Input: part model. Units: mm. Frame: model coordinates. A direction names the side the tool comes from. Give positions to 0.01 mm unless a question says otherwise; leave off trailing zeros. Loops run counter-clockwise (first coordinate to the right, second up) from the corner with the lowest first, then second, coordinate; pieces in that order, holes last. Notation, with made-up numbers: (51.5, 7) - (93.5, 7) arc R22 cw to (93.5, 30) - close; hole circle Ø8 at (27.25, 57). An arc over 180 degrees is marked (long way). Answer as a JSON object with one key per item and string values. Group by question number.
(1) Mould query, pull axis Z, two halves, no side actions, for faces 1 (the flat face through (0, 8, 9)), 2 (the flat face through (0, 2, -25.981)), 3 (the cylindrical face through (1.008, 1.423, 31.078)). Classes: +Z half, -Z half, draft (parallel to the pull), parting line (faces both ways), or undercut.
(2) Section query B-B (z = 17). Return loops of the section in (x, y), plus the area to 3 significant figures.
(3) Pin query (flat end, axial travel): P1, Ø2, axis at y = 3.5, z = -14, coming from the -X side; P2, Ø2, axis at y = 1.5, z = -8.5, coming from the -X side; P3, Ø4, axis at x = -30.5, y = 4.5, coming from the +Z side; P4, Ø4, axis at y = 1, z = -10.5, coming from the +X side. Return the tip coordinate at first contact, or that it passes through.
(4) Access query for faces 4 (the cylindrical face through (-22.624, 4.056, -13.77)), 5 (the cylindrical face through (-6.967, 6.768, 4.229)). Directions: +Z, -Z, +X, -X, +Y, -Y. A direction counts if a zero-diameter tool reaches every point of the face in a straight line with its end or side. Return the directions, or none.
(5) Material intervals for L1, parallel to Z at x = -27.5, y = 3.5; L2, parallel to X at y = 3, z = 9; L3, parallel to Z at x = 17, y = 3.5, sorted ascending.
(6) Section query A-A (z = 0). Return loops of the section in (x, y), plus the area to 3 significant figures.
```python
from build123d import *

# Parameters (mm, degrees)
BOSS_EXTRUDE1_DEPTH   = 8
CHAMFER1_SIZE         = 4
CHAMFER1_SIZE2        = 6.928203
CHAMFER1_PART_2_SIZE  = 4
CHAMFER1_PART_2_SIZE2 = 6.928203
CHAMFER1_PART_3_SIZE  = 4
CHAMFER1_PART_3_SIZE2 = 6.928203
CUT_EXTRUDE1_REACH    = 61.292
SKETCH2_R             = 1.6
CUT_EXTRUDE2_REACH    = 67.292
CUT_EXTRUDE2_START    = -6
SKETCH3_R             = 3
CIRPATTERN1_COUNT     = 3
CUT_EXTRUDE4_DEPTH    = 2.5
CUT_EXTRUDE5_REACH    = 57.633
SKETCH10_R            = 1.6


with BuildPart() as part:
    # Sketch1 → Boss-Extrude1 (new body)
    with BuildSketch(Plane(origin=(0, 0, 0), x_dir=(1, 0, 0), z_dir=(0, 1, 0))):
        Polygon((-31, 25.980762), (31, 25.980762), (38, 13.856406), (7, -39.837169), (-7, -39.837169), (-38, 13.856406), align=None)
        with BuildLine():
            Line((3.923683, -4.605129), (5.655734, -3.605129))
            ThreePointArc((5.655734, -3.605129), (14.562222, 8.407503), (-0.294266, 6.700574))
            Line((-0.294266, 6.700574), (-2.026317, 5.700574))
            ThreePointArc((-2.026317, 5.700574), (-5.239454, -3.025), (3.923683, -4.605129))
        make_face(mode=Mode.SUBTRACT)
    extrude(amount=BOSS_EXTRUDE1_DEPTH)

    # Chamfer1
    chamfer1_edges = [part.edges().sort_by_distance(p)[0] for p in [
        (22.5, 8, 12.990381),
    ]]
    chamfer1_side = [part.faces().sort_by_distance(p)[0] for p in [
        (22.5, 4, 12.990381),
    ]]
    chamfer(chamfer1_edges, length=CHAMFER1_SIZE, length2=CHAMFER1_SIZE2, reference=chamfer1_side[0])

    # Chamfer1 part 2
    chamfer1_part_2_edges = [part.edges().sort_by_distance(p)[0] for p in [
        (-22.5, 8, 12.990381),
    ]]
    chamfer1_part_2_side = [part.faces().sort_by_distance(p)[0] for p in [
        (-22.5, 4, 12.990381),
    ]]
    chamfer(chamfer1_part_2_edges, length=CHAMFER1_PART_2_SIZE, length2=CHAMFER1_PART_2_SIZE2, reference=chamfer1_part_2_side[0])

    # Chamfer1 part 3
    chamfer1_part_3_edges = [part.edges().sort_by_distance(p)[0] for p in [
        (0, 8, -25.980762),
    ]]
    chamfer1_part_3_side = [part.faces().sort_by_distance(p)[0] for p in [
        (0, 4, -25.980762),
    ]]
    chamfer(chamfer1_part_3_edges, length=CHAMFER1_PART_3_SIZE, length2=CHAMFER1_PART_3_SIZE2, reference=chamfer1_part_3_side[0])

    # Cut-Extrude1: up to this plane
    cut_extrude1_end = Plane(origin=(0, 0, 0), z_dir=(0, -1, 0))
    # Sketch2 → Cut-Extrude1 (cut, up to the surface)
    with BuildSketch(Plane(origin=(7.125, 14.25, 4.113621), x_dir=(0.9013878188659966, -0.41602514716892336, -0.12009611535381544), z_dir=(0.43301270189222085, 0.8660254037844383, 0.24999999999999917)), mode=Mode.PRIVATE) as cut_extrude1_sk1:
        with Locations(Location((28.428385, 12.89678, 0), (0, 0, 172.874984))):
            Circle(SKETCH2_R)
    cut_extrude1_tool1 = split(extrude(cut_extrude1_sk1.sketch, amount=-CUT_EXTRUDE1_REACH, mode=Mode.PRIVATE), bisect_by=cut_extrude1_end, keep=Keep.BOTH, mode=Mode.PRIVATE)
    # Sketch2 → Cut-Extrude1 (cut, up to the surface)
    with BuildSketch(Plane(origin=(7.125, 14.25, 4.113621), x_dir=(0.9013878188659966, -0.41602514716892336, -0.12009611535381544), z_dir=(0.43301270189222085, 0.8660254037844383, 0.24999999999999917)), mode=Mode.PRIVATE) as cut_extrude1_sk2:
        with Locations(Location((-0.970725, -31.201886, 0), (0, 0, 172.874984))):
            Circle(SKETCH2_R)
    cut_extrude1_tool2 = split(extrude(cut_extrude1_sk2.sketch, amount=-CUT_EXTRUDE1_REACH, mode=Mode.PRIVATE), bisect_by=cut_extrude1_end, keep=Keep.BOTH, mode=Mode.PRIVATE)
    # Sketch2 → Cut-Extrude1 (cut, up to the surface)
    with BuildSketch(Plane(origin=(7.125, 14.25, 4.113621), x_dir=(0.9013878188659966, -0.41602514716892336, -0.12009611535381544), z_dir=(0.43301270189222085, 0.8660254037844383, 0.24999999999999917)), mode=Mode.PRIVATE) as cut_extrude1_sk3:
        with Locations(Location((13.72883, -9.152553, 0), (0, 0, 172.874984))):
            Circle(SKETCH2_R)
    cut_extrude1_tool3 = split(extrude(cut_extrude1_sk3.sketch, amount=-CUT_EXTRUDE1_REACH, mode=Mode.PRIVATE), bisect_by=cut_extrude1_end, keep=Keep.BOTH, mode=Mode.PRIVATE)
    # Sketch2 → Cut-Extrude1 (cut, up to the surface)
    with BuildSketch(Plane(origin=(7.125, 14.25, 4.113621), x_dir=(0.9013878188659966, -0.41602514716892336, -0.12009611535381544), z_dir=(0.43301270189222085, 0.8660254037844383, 0.24999999999999917)), mode=Mode.PRIVATE) as cut_extrude1_sk4:
        with Locations(Location((22.881383, 4.576277, 0), (0, 0, 172.874984))):
            Circle(SKETCH2_R)
    cut_extrude1_tool4 = split(extrude(cut_extrude1_sk4.sketch, amount=-CUT_EXTRUDE1_REACH, mode=Mode.PRIVATE), bisect_by=cut_extrude1_end, keep=Keep.BOTH, mode=Mode.PRIVATE)
    # Sketch2 → Cut-Extrude1 (cut, up to the surface)
    with BuildSketch(Plane(origin=(7.125, 14.25, 4.113621), x_dir=(0.9013878188659966, -0.41602514716892336, -0.12009611535381544), z_dir=(0.43301270189222085, 0.8660254037844383, 0.24999999999999917)), mode=Mode.PRIVATE) as cut_extrude1_sk5:
        with Locations(Location((4.576277, -22.881383, 0), (0, 0, 172.874984))):
            Circle(SKETCH2_R)
    cut_extrude1_tool5 = split(extrude(cut_extrude1_sk5.sketch, amount=-CUT_EXTRUDE1_REACH, mode=Mode.PRIVATE), bisect_by=cut_extrude1_end, keep=Keep.BOTH, mode=Mode.PRIVATE)
    cut_extrude1 = cut_extrude1_tool1.solids().sort_by_distance((32.75, 6, -11.691343))[0] + cut_extrude1_tool2.solids().sort_by_distance((6.25, 6, 34.208003))[0] + cut_extrude1_tool3.solids().sort_by_distance((19.5, 6, 11.25833))[0] + cut_extrude1_tool4.solids().sort_by_distance((27.75, 6, -3.031089))[0] + cut_extrude1_tool5.solids().sort_by_distance((11.25, 6, 25.547749))[0]
    add(cut_extrude1, mode=Mode.SUBTRACT)

    # Sketch3 → Cut-Extrude2 (cut, up to next)
    with BuildSketch(Plane(origin=(7.125, 14.25, 4.113621), x_dir=(0.9013878188659967, -0.41602514716892325, -0.12009611535381544), z_dir=(0.43301270189222074, 0.8660254037844383, 0.24999999999999925)).offset(CUT_EXTRUDE2_START), mode=Mode.PRIVATE) as cut_extrude2_sk1:
        with Locations((28.428385, 12.89678)):
            Circle(SKETCH3_R)
    cut_extrude2_tool1 = extrude(cut_extrude2_sk1.sketch, amount=-CUT_EXTRUDE2_REACH, mode=Mode.PRIVATE) & part.part
    # Sketch3 → Cut-Extrude2 (cut, up to next)
    with BuildSketch(Plane(origin=(7.125, 14.25, 4.113621), x_dir=(0.9013878188659967, -0.41602514716892325, -0.12009611535381544), z_dir=(0.43301270189222074, 0.8660254037844383, 0.24999999999999925)).offset(CUT_EXTRUDE2_START), mode=Mode.PRIVATE) as cut_extrude2_sk2:
        with Locations((-0.970725, -31.201886)):
            Circle(SKETCH3_R)
    cut_extrude2_tool2 = extrude(cut_extrude2_sk2.sketch, amount=-CUT_EXTRUDE2_REACH, mode=Mode.PRIVATE) & part.part
    # Sketch3 → Cut-Extrude2 (cut, up to next)
    with BuildSketch(Plane(origin=(7.125, 14.25, 4.113621), x_dir=(0.9013878188659967, -0.41602514716892325, -0.12009611535381544), z_dir=(0.43301270189222074, 0.8660254037844383, 0.24999999999999925)).offset(CUT_EXTRUDE2_START), mode=Mode.PRIVATE) as cut_extrude2_sk3:
        with Locations((13.72883, -9.152553)):
            Circle(SKETCH3_R)
    cut_extrude2_tool3 = extrude(cut_extrude2_sk3.sketch, amount=-CUT_EXTRUDE2_REACH, mode=Mode.PRIVATE) & part.part
    # Sketch3 → Cut-Extrude2 (cut, up to next)
    with BuildSketch(Plane(origin=(7.125, 14.25, 4.113621), x_dir=(0.9013878188659967, -0.41602514716892325, -0.12009611535381544), z_dir=(0.43301270189222074, 0.8660254037844383, 0.24999999999999925)).offset(CUT_EXTRUDE2_START), mode=Mode.PRIVATE) as cut_extrude2_sk4:
        with Locations((22.881383, 4.576277)):
            Circle(SKETCH3_R)
    cut_extrude2_tool4 = extrude(cut_extrude2_sk4.sketch, amount=-CUT_EXTRUDE2_REACH, mode=Mode.PRIVATE) & part.part
    # Sketch3 → Cut-Extrude2 (cut, up to next)
    with BuildSketch(Plane(origin=(7.125, 14.25, 4.113621), x_dir=(0.9013878188659967, -0.41602514716892325, -0.12009611535381544), z_dir=(0.43301270189222074, 0.8660254037844383, 0.24999999999999925)).offset(CUT_EXTRUDE2_START), mode=Mode.PRIVATE) as cut_extrude2_sk5:
        with Locations((4.576277, -22.881383)):
            Circle(SKETCH3_R)
    cut_extrude2_tool5 = extrude(cut_extrude2_sk5.sketch, amount=-CUT_EXTRUDE2_REACH, mode=Mode.PRIVATE) & part.part
    cut_extrude2_1 = cut_extrude2_tool1.solids().sort_by_distance((30.151924, 0.803848, -13.191343))[0]
    add(cut_extrude2_1, mode=Mode.SUBTRACT)
    cut_extrude2_2 = cut_extrude2_tool2.solids().sort_by_distance((3.651924, 0.803848, 32.708003))[0]
    add(cut_extrude2_2, mode=Mode.SUBTRACT)
    cut_extrude2_3 = cut_extrude2_tool3.solids().sort_by_distance((16.901924, 0.803848, 9.75833))[0]
    add(cut_extrude2_3, mode=Mode.SUBTRACT)
    cut_extrude2_4 = cut_extrude2_tool4.solids().sort_by_distance((25.151924, 0.803848, -4.531089))[0]
    add(cut_extrude2_4, mode=Mode.SUBTRACT)
    cut_extrude2_5 = cut_extrude2_tool5.solids().sort_by_distance((8.651924, 0.803848, 24.047749))[0]
    add(cut_extrude2_5, mode=Mode.SUBTRACT)
    cut_extrude2 = cut_extrude2_1 + cut_extrude2_2 + cut_extrude2_3 + cut_extrude2_4 + cut_extrude2_5  # Cut-Extrude2 as one shape, for the pattern or mirror that repeats it

    # CirPattern1: Cut-Extrude1, Cut-Extrude2 ×3 about axis
    cirpattern1_axis = Axis((0, 0, 0), (0, 1, 0))
    add([cut_extrude1.rotate(cirpattern1_axis, i * 360 / CIRPATTERN1_COUNT) for i in range(1, CIRPATTERN1_COUNT)], mode=Mode.SUBTRACT)
    add([cut_extrude2.rotate(cirpattern1_axis, i * 360 / CIRPATTERN1_COUNT) for i in range(1, CIRPATTERN1_COUNT)], mode=Mode.SUBTRACT)

    # Sketch8 → Cut-Extrude4 (cut)
    with BuildSketch(Plane(origin=(0, 8, 0), x_dir=(1, 0, 0), z_dir=(0, 1, 0))):
        with BuildLine():
            Line((-4.075, 7.058107), (3.429115, 11.39061))
            ThreePointArc((3.429115, 11.39061), (14.562222, 8.407503), (11.579115, -2.725604))
            Line((11.579115, -2.725604), (4.075, -7.058107))
            ThreePointArc((4.075, -7.058107), (-7.058107, -4.075), (-4.075, 7.058107))
        make_face()
    extrude(amount=-CUT_EXTRUDE4_DEPTH, mode=Mode.SUBTRACT)

    # Sketch10 → Cut-Extrude5 (cut, up to next)
    with BuildSketch(Plane(origin=(0, 8, 0), x_dir=(1, 0, 0), z_dir=(0, 1, 0)), mode=Mode.PRIVATE) as cut_extrude5_sk1:
        with Locations(Location((21.650635, 12.5, 0), (0, 0, 270))):
            Circle(SKETCH10_R)
    cut_extrude5_tool1 = extrude(cut_extrude5_sk1.sketch, amount=-CUT_EXTRUDE5_REACH, mode=Mode.PRIVATE) & part.part
    # Sketch10 → Cut-Extrude5 (cut, up to next)
    with BuildSketch(Plane(origin=(0, 8, 0), x_dir=(1, 0, 0), z_dir=(0, 1, 0)), mode=Mode.PRIVATE) as cut_extrude5_sk2:
        with Locations(Location((0, -25, 0), (0, 0, 270))):
            Circle(SKETCH10_R)
    cut_extrude5_tool2 = extrude(cut_extrude5_sk2.sketch, amount=-CUT_EXTRUDE5_REACH, mode=Mode.PRIVATE) & part.part
    # Sketch10 → Cut-Extrude5 (cut, up to next)
    with BuildSketch(Plane(origin=(0, 8, 0), x_dir=(1, 0, 0), z_dir=(0, 1, 0)), mode=Mode.PRIVATE) as cut_extrude5_sk3:
        with Locations(Location((-21.650635, 12.5, 0), (0, 0, 270))):
            Circle(SKETCH10_R)
    cut_extrude5_tool3 = extrude(cut_extrude5_sk3.sketch, amount=-CUT_EXTRUDE5_REACH, mode=Mode.PRIVATE) & part.part
    add(cut_extrude5_tool1.solids().sort_by_distance((21.650635, 8, -12.5))[0], mode=Mode.SUBTRACT)
    add(cut_extrude5_tool2.solids().sort_by_distance((0, 8, 25))[0], mode=Mode.SUBTRACT)
    add(cut_extrude5_tool3.solids().sort_by_distance((-21.650635, 8, -12.5))[0], mode=Mode.SUBTRACT)


solid = part.part
```
Recorded:
{
 "1": {"face 1": "draft", "face 2": "-Z half", "face 3": "undercut"},
 "2": {"outline": "(-20.19, 0) - (20.19, 0) - (20.19, 4) - (12.19, 8) - (-12.19, 8) - (-20.19, 4) - close", "area": "291 mm^2"},
 "3": {"P1": "stops at x = -38", "P2": "stops at x = -35.48", "P3": "stops at z = 2.49", "P4": "stops at x = 37.22"},
 "4": {"face 4": "+Y, -Y", "face 5": "+Y"},
 "5": {"L1": "z = -25.98 to -22.52, -19.63 to -5.01, -2.27 to 4.33", "L2": "x = -24.8 to -18.79, -16.84 to 16.84, 18.79 to 24.8", "L3": "z = -25.98 to -22.83, -19.32 to 9.21, 11.57 to 22.52"},
 "6": {"outline": "(-30, 0) - (-6.05, 0) - (-6.05, 5.5) - (-8.15, 5.5) - (-8.15, 8) - (-22, 8) - (-30, 4) - close; (14.41, 0) - (30, 0) - (30, 4) - (22, 8) - (14.41, 8) - close", "area": "279 mm^2"}
}
